```python
from build123d import *

# Parameters (mm, degrees)
F0_R     = 2.15265
F0_R_2   = 14.2875
F1_DEPTH = 8.89
F2_R     = 2.15265
F2_R_2   = 14.2875
F2_R_3   = 12.7
F3_DEPTH = 3.175


with BuildPart() as f1:
    # F0 (on Top) → F1 (new body)
    with BuildSketch(Plane.XY):
        with BuildLine():
            Line((3.96875, 17.0055264455), (3.96875, 18.25625))
            ThreePointArc((3.96875, 18.25625), (0, 22.225), (-3.96875, 18.25625))
            Line((-3.96875, 18.25625), (-3.96875, 17.0055264455))
            ThreePointArc((-3.96875, 17.0055264455), (-12.3478521665, 12.3478521665), (-17.0055264455, 3.96875))
            Line((-17.0055264455, 3.96875), (-18.25625, 3.96875))
            ThreePointArc((-18.25625, 3.96875), (-22.225, 0), (-18.25625, -3.96875))
            Line((-18.25625, -3.96875), (-17.0055264455, -3.96875))
            ThreePointArc((-17.0055264455, -3.96875), (-12.3478521665, -12.3478521665), (-3.96875, -17.0055264455))
            Line((-3.96875, -17.0055264455), (-3.96875, -18.25625))
            ThreePointArc((-3.96875, -18.25625), (0, -22.225), (3.96875, -18.25625))
            Line((3.96875, -18.25625), (3.96875, -17.0055264455))
            ThreePointArc((3.96875, -17.0055264455), (12.3478521665, -12.3478521665), (17.0055264455, -3.96875))
            Line((17.0055264455, -3.96875), (18.25625, -3.96875))
            ThreePointArc((18.25625, -3.96875), (22.225, 0), (18.25625, 3.96875))
            Line((18.25625, 3.96875), (17.0055264455, 3.96875))
            ThreePointArc((17.0055264455, 3.96875), (12.3478521665, 12.3478521665), (3.96875, 17.0055264455))
        make_face()
        with Locations((0, -18.25625)):
            Circle(F0_R, mode=Mode.SUBTRACT)
        with Locations((-18.25625, 0)):
            Circle(F0_R, mode=Mode.SUBTRACT)
        Circle(F0_R_2, mode=Mode.SUBTRACT)
        with Locations((18.25625, 0)):
            Circle(F0_R, mode=Mode.SUBTRACT)
        with Locations((0, 18.25625)):
            Circle(F0_R, mode=Mode.SUBTRACT)
    extrude(amount=F1_DEPTH)

    # F2 (on face) → F3 (join)
    with BuildSketch(Plane.XY.offset(8.89)):
        with BuildLine():
            ThreePointArc((-17.0055264455, -3.96875), (-12.3478521665, -12.3478521665), (-3.96875, -17.0055264455))
            Line((-3.96875, -17.0055264455), (-3.96875, -18.25625))
            ThreePointArc((-3.96875, -18.25625), (0, -22.225), (3.96875, -18.25625))
            Line((3.96875, -18.25625), (3.96875, -17.0055264455))
            ThreePointArc((3.96875, -17.0055264455), (12.3478521665, -12.3478521665), (17.0055264455, -3.96875))
            Line((17.0055264455, -3.96875), (18.25625, -3.96875))
            ThreePointArc((18.25625, -3.96875), (22.225, 0), (18.25625, 3.96875))
            Line((18.25625, 3.96875), (17.0055264455, 3.96875))
            ThreePointArc((17.0055264455, 3.96875), (12.3478521665, 12.3478521665), (3.96875, 17.0055264455))
            Line((3.96875, 17.0055264455), (3.96875, 18.25625))
            ThreePointArc((3.96875, 18.25625), (0, 22.225), (-3.96875, 18.25625))
            Line((-3.96875, 18.25625), (-3.96875, 17.0055264455))
            ThreePointArc((-3.96875, 17.0055264455), (-12.3478521665, 12.3478521665), (-17.0055264455, 3.96875))
            Line((-17.0055264455, 3.96875), (-18.25625, 3.96875))
            ThreePointArc((-18.25625, 3.96875), (-22.225, 0), (-18.25625, -3.96875))
            Line((-18.25625, -3.96875), (-17.0055264455, -3.96875))
        make_face()
        with Locations((0, -18.25625)):
            Circle(F2_R, mode=Mode.SUBTRACT)
        with Locations((-18.25625, 0)):
            Circle(F2_R, mode=Mode.SUBTRACT)
        Circle(F2_R_2, mode=Mode.SUBTRACT)
        with Locations((18.25625, 0)):
            Circle(F2_R, mode=Mode.SUBTRACT)
        with Locations((0, 18.25625)):
            Circle(F2_R, mode=Mode.SUBTRACT)
        Circle(F2_R_2)
        Circle(F2_R_3, mode=Mode.SUBTRACT)
    extrude(amount=F3_DEPTH)


solid = f1.part
```
Part model, mm, in its own coordinate system. A direction names the side the tool comes from. Give positions to 0.01 mm unless a question says otherwise; leave off trailing zeros. Loops run counter-clockwise (first coordinate to the right, second up) from the corner with the lowest first, then second, coordinate; pieces in that order, holes last. Notation, with made-up numbers: M -38,43 L -13,43 A10 ccw -13,55 Z; hole C 38,64 d7. An arc over 180 degrees is marked long. Return JSON: item names as keys, results as strings.
1) Saw through at D-D, the plane x = 5.5. List the corners of the cut face in (y, z) (3 decimals), then the cut area to 3 significant figures.
Calculated:
{"outline": "M -16.574,0 L -13.186,0 L -13.186,8.89 L -11.447,8.89 L -11.447,12.065 L -16.574,12.065 Z; M 11.447,8.89 L 13.186,8.89 L 13.186,0 L 16.574,0 L 16.574,12.065 L 11.447,12.065 Z", "area": "92.8 mm2"}
2) Saw through at A-A, the plane z = 10.25. List the corners of the cut face in (x, y) (1 decimal).
Calculated:
{"outline": "M -18.3,-4 L -17,-4 A17.5 ccw -4,-17 L -4,-18.3 A4 ccw 4,-18.3 L 4,-17 A17.5 ccw 17,-4 L 18.3,-4 A4 ccw 18.3,4 L 17,4 A17.5 ccw 4,17 L 4,18.3 A4 ccw -4,18.3 L -4,17 A17.5 ccw -17,4 L -18.3,4 A4 ccw Z; hole C -18.3,0 d4.3; hole C 0,0 d25.4; hole C 0,-18.3 d4.3; hole C 0,18.3 d4.3; hole C 18.3,0 d4.3"}
3) 3-axis set-ups, long thin cutter, end or side, ignore diameter. For faces 1 (the face through (-2.75, -12.4, 10.46)), 2 (the face through (-14.274, 0.628, 4.383)), 3 (the face through (3.969, 18, 6)), 4 (the face through (-3.969, 18, 6)), 5 (the face through (3.969, -18, 6)): which of +Z, -Z, +X, -X, +Y, -Y reach the whole face in a straight line?
Calculated:
{"face 1": "+Z, -Z", "face 2": "-Z", "face 3": "+Z, -Z, +X, +Y", "face 4": "+Z, -Z, -X, +Y", "face 5": "+Z, -Z, +X, -Y"}
4) Flat gauge pins, fed straight in: pin 1 Ø5 at (x, y) = (0.5, -15) entering from -Z; pin 2 Ø4 at (y, z) = (16, 9.5) entering from -X; pin 3 Ø1 at (y, z) = (-3, 2) entering from +X; pin 4 Ø3 at (x, z) = (9, 7) entering from -Y. Where does each tip first touch, or does it go through?
Calculated:
{"pin 1": "stops at z = 0", "pin 2": "stops at x = -10.44", "pin 3": "stops at x = 21.34", "pin 4": "stops at y = -15.77"}
5) Pull direction X, two halves, no side cores. Call faces 6 (the face through (0.993, 16.346, 5.948)), 7 (the face through (0.993, -20.166, 5.948)), 8 (the face through (-18, -3.969, 6)), 9 (the face through (-12.444, -12.251, 5.948)): released by +X, released by -X, zero draft, split by the parting line, or undercut.
Calculated:
{"face 6": "undercut", "face 7": "undercut", "face 8": "zero draft", "face 9": "released by -X"}
6) Drill centre lines: line 1 (Y direction, x = 0, z = 7.25) (1 decimal); line 2 (X direction, y = 8.5, z = 9.5); line 3 (X direction, y = 1, z = 4.75). Where is each one in solid material? Low to high.
Calculated:
{"line 1": "y = -22.2 to -20.4, -16.1 to -14.3, 14.3 to 16.1, 20.4 to 22.2", "line 2": "x = -15.25 to -9.44, 9.44 to 15.25", "line 3": "x = -22.1 to -20.16, -16.35 to -14.25, 14.25 to 16.35, 20.16 to 22.1"}
7) Saw through at B-B, the plane y = 0. List the corners of the cut face in (x, z) (1 decimal).
Calculated:
{"outline": "M -22.2,0 L -20.4,0 L -20.4,12.1 L -22.2,12.1 Z; M -16.1,0 L -14.3,0 L -14.3,8.9 L -12.7,8.9 L -12.7,12.1 L -16.1,12.1 Z; M 12.7,8.9 L 14.3,8.9 L 14.3,0 L 16.1,0 L 16.1,12.1 L 12.7,12.1 Z; M 20.4,0 L 22.2,0 L 22.2,12.1 L 20.4,12.1 Z"}
